Solid Edge part; units mm, degrees
sketch "Sketch1" plane through (0, 0, 0) normal (0, -1, 0) x (1, 0, 0)
  line L0 (125, 60) -> (0, 60)
  line L1 (0, 60) -> (0, 0)
  line L2 (0, 0) -> (125, 0)
  line L3 (125, 0) -> (125, 60)
extrude "Protrusion1" add sketch "Sketch1" against normal blind 90
sketch "Sketch2" plane through (125, 45, 30) normal (1, 0, 0) x (0, 1, 0)
  line L0 (-45, -10) -> (-45, 30)
  line L1 (-45, 30) -> (15, 30)
  line L2 (15, 30) -> (15, 10)
  line L3 (15, 10) -> (-15, 10)
  line L4 (-15, 10) -> (-15, -10)
  line L5 (-15, -10) -> (-45, -10)
extrude "ExtrudedCutout_1" cut sketch "Sketch2" against normal blind 80
The model under review builds one solid part; all positions refer to its coordinate system, in mm. A direction names the side the tool comes from. Coordinates: 2 decimals unless noted, no trailing zeros. Loops run counter-clockwise (first coordinate to the right, second up) from the corner with the lowest first, then second, coordinate; pieces in that order, holes last.
(1) Draft analysis for pull direction Y (two halves, no side actions). For faces 1 (the flat face through (49, 0, 17)), 2 (the flat face through (63, 90, 30)), 3 (the flat face through (45, 23, 45)), state which applies: +Y half, -Y half, draft (parallel to the pull), parting line (faces both ways), or undercut.
Determined:
face 1: -Y half
face 2: +Y half
face 3: draft
(2) Tool access review of faces 4 (the flat face through (0, 44, 30)), 5 (the flat face through (86, 30, 30)): name each direction out of +Z, -Z, +X, -X, +Y, -Y from which nothing blocks a thin tool from reaching the whole face with its end or side.
Determined:
face 4: +Z, -Z, -X, +Y, -Y
face 5: +Z, +X, -Y
(3) Consider section A-A, the plane z = 32. Give the boundary of the cut face in (x, y), plus the area to 3 significant figures.
Determined:
outline: (0, 0) - (45, 0) - (45, 30) - (125, 30) - (125, 90) - (0, 90) - close
area: 8,850 mm2
(4) Consider section C-C, the plane x = 113. Give the boundary of the cut face in (y, z), plus the area to 3 significant figures.
Determined:
outline: (0, 0) - (90, 0) - (90, 60) - (60, 60) - (60, 40) - (30, 40) - (30, 20) - (0, 20) - close
area: 3,600 mm2
(5) Insertion check: P1, Ø15, axis at x = 101, y = 50.5, coming from the +Z side; P2, Ø4, axis at y = 47.5, z = 51.5, coming from the +X side; P3, Ø22, axis at x = 93, z = 47.5, coming from the -Y side. Each pin has a flat end and moves straight along its axis. Give the tip position at first contact, or say it passes through.
Determined:
P1: stops at z = 40
P2: stops at x = 45
P3: stops at y = 30
(6) Wall thickness on L1, parallel to Z at x = 94.5, y = 27.5; L2, parallel to Y at x = 76, z = 34; L3, parallel to Y at x = 64, z = 43: over which ranges is each line inside the solid? List them lowest first.
Determined:
L1: z = 0 to 20
L2: y = 30 to 90
L3: y = 60 to 90
(7) Consider section B-B, the plane y = 38. Give the boundary of the cut face in (x, z).
Determined:
outline: (0, 0) - (125, 0) - (125, 40) - (45, 40) - (45, 60) - (0, 60) - close
